from build123d import *

# Parameters (mm, degrees)
ESQUISSE1_R        = 1.5
BOSS_EXTRU_2_DEPTH = 6


with BuildPart() as part:
    # Esquisse1 → Boss.-Extru.2 (new body)
    with BuildSketch(Plane.XY):
        with BuildLine():
            ThreePointArc((-2.411034891, 11.820685714), (0, 10.75), (2.411034891, 11.820685714))
            ThreePointArc((2.411034891, 11.820685714), (3.975330286, 12.779130538), (5.80943088, 12.737759334))
            ThreePointArc((5.80943088, 12.737759334), (11.865562564, 7.430237213), (13.995977593, -0.335575935))
            ThreePointArc((13.995977593, -0.335575935), (13.382779595, -2.564868949), (11.442531564, -3.822325392))
            ThreePointArc((11.442531564, -3.822325392), (9.309773091, -5.375), (9.031496673, -7.998360322))
            ThreePointArc((9.031496673, -7.998360322), (9.079386541, -9.832302285), (8.126507731, -11.399994391))
            ThreePointArc((8.126507731, -11.399994391), (0.5019929, -13.990997217), (-7.288606081, -11.953084179))
            ThreePointArc((-7.288606081, -11.953084179), (-8.912631465, -10.307392628), (-9.031496673, -7.998360322))
            ThreePointArc((-9.031496673, -7.998360322), (-9.309773091, -5.375), (-11.442531564, -3.822325392))
            ThreePointArc((-11.442531564, -3.822325392), (-13.054716827, -2.946828253), (-13.935938611, -1.337764944))
            ThreePointArc((-13.935938611, -1.337764944), (-12.367555464, 6.560760004), (-6.707371512, 12.288660114))
            ThreePointArc((-6.707371512, 12.288660114), (-4.47014813, 12.872261577), (-2.411034891, 11.820685714))
        make_face()
        with Locations((9.526279442, 5.5)):
            Circle(ESQUISSE1_R, mode=Mode.SUBTRACT)
        with Locations((0, -11)):
            Circle(ESQUISSE1_R, mode=Mode.SUBTRACT)
        with Locations((-9.526279442, 5.5)):
            Circle(ESQUISSE1_R, mode=Mode.SUBTRACT)
    extrude(amount=BOSS_EXTRU_2_DEPTH)


solid = part.part
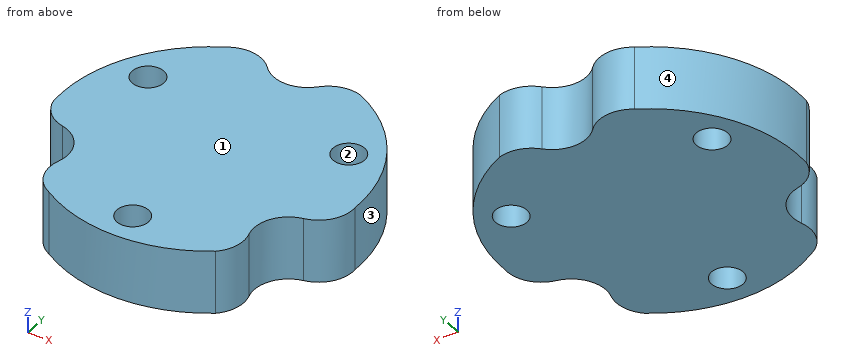
Model file for the job. Use its own axes, mm. Face numbers are marked on the shaded views. Round coordinates to 2 decimals unless told otherwise and drop trailing zeros. Loops run counter-clockwise (first coordinate to the right, second up) from the corner with the lowest first, then second, coordinate; pieces in that order, holes last.
1. Band-saw the part on C-C, the plane z = 4.55. List the corners of the cut face in (x, y).
Check values:
outline: (-13.94, -1.34) arc R3.25 ccw to (-11.44, -3.82) arc R3.25 cw to (-9.03, -8) arc R3.25 ccw to (-7.29, -11.95) arc R14 ccw to (8.13, -11.4) arc R3.25 ccw to (9.03, -8) arc R3.25 cw to (11.44, -3.82) arc R3.25 ccw to (14, -0.34) arc R14 ccw to (5.81, 12.74) arc R3.25 ccw to (2.41, 11.82) arc R3.25 cw to (-2.41, 11.82) arc R3.25 ccw to (-6.71, 12.29) arc R14 ccw to start; hole circle Ø3 at (-9.53, 5.5); hole circle Ø3 at (0, -11); hole circle Ø3 at (9.53, 5.5)
2. Band-saw the part on A-A, the plane x = 0. List the corners of the cut face in (y, z), and give its area (4 significant figures).
Check values:
outline: (-14, 0) - (-12.5, 0) - (-12.5, 6) - (-14, 6) - close; (-9.5, 0) - (10.75, 0) - (10.75, 6) - (-9.5, 6) - close
area: 130.5 mm2
3. Mould opens along X. For the marked faces 1, 2, 3 and 4 say: +X half, -X half, draft (parallel to the pull), parting line (faces both ways), or undercut.
Check values:
face 1: draft
face 2: undercut
face 3: +X half
face 4: -X half
4. Drop a flat-ended pin along its axis: P1, Ø1.5, axis at y = 6, z = 2, coming from the -X side. Give the stop position or say it passes through.
Check values:
P1: stops at x = -12.98
5. Wall check: probe 1 along Y at (x, z) = (0, 4.8); probe 2 along X at (y, z) = (6.25, 4.9); probe 3 along X at (y, z) = (-11.5, 4.6). Give the ranges that are in metal, low to high.
Check values:
probe 1: y = -14 to -12.5, -9.5 to 10.75
probe 2: x = -12.53 to -10.83, -8.23 to 8.23, 10.83 to 12.53
probe 3: x = -8.01 to -1.41, 1.41 to 7.98
6. Band-saw the part on D-D, the plane y = 5.5. List the corners of the cut face in (x, z).
Check values:
outline: (-12.87, 0) - (-11.03, 0) - (-11.03, 6) - (-12.87, 6) - close; (-8.03, 0) - (8.03, 0) - (8.03, 6) - (-8.03, 6) - close; (11.03, 0) - (12.87, 0) - (12.87, 6) - (11.03, 6) - close
7. Band-saw the part on B-B, the plane y = -11. List the corners of the cut face in (x, z), and give its area (3 significant figures).
Check values:
outline: (-8.5, 0) - (-1.5, 0) - (-1.5, 6) - (-8.5, 6) - close; (1.5, 0) - (8.5, 0) - (8.5, 6) - (1.5, 6) - close
area: 84.0 mm2
